Autodesk Inventor part; units mm, degrees
ref_plane "ip_st_1_XY" through (0, 0, 0) normal (1, 0, 0) x (0, 0, -1)
ref_plane "ip_st_1_YZ" through (0, 0, 0) normal (0, 0, -1) x (0, 1, 0)
ref_plane "ip_st_1_ZX" through (0, 0, 0) normal (0, 1, 0) x (1, 0, 0)
sketch "Sketch_1" plane through (0, 0, 0) normal (0, 0, 1) x (1, 0, 0)
  line L0 (4, 0) -> (0, 0)
  line L1 (0, 4.925) -> (0.25, 4.925)
  line L2 (0.25, 4.925) -> (0.25, 4.475)
  line L3 (0.25, 4.475) -> (1.2405, 4.475)
  arc A0 (2.7595, 4.475) -> (1.2405, 4.475) centre (2, 3.75) ccw
  line L4 (2.7595, 4.475) -> (3.75, 4.475)
  line L5 (3.75, 4.475) -> (3.75, 4.925)
  line L6 (3.75, 4.925) -> (4, 4.925)
  line L7 (4, 4.925) -> (4, 6.1)
  arc A1 (4, 6.1) -> (3.85, 6.25) centre (3.85, 6.1) ccw
  line L8 (3.85, 6.25) -> (3, 6.25)
  line L9 (3, 6.25) -> (3, 5.5)
  line L10 (3, 5.5) -> (0.15, 5.5)
  arc A2 (0.15, 5.5) -> (0, 5.35) centre (0.15, 5.35) ccw
  line L11 (0, 5.35) -> (0, 4.925)
revolve "Revolution1" add sketch "Sketch_1" angle 360 about axis through (4, 0, 0) along (1, 0, 0)
ref_plane "ip_st_1_XY" through (0, 0, 0) normal (1, 0, 0) x (0, 0, -1)
ref_plane "ip_st_1_YZ" through (0, 0, 0) normal (0, 0, -1) x (0, 1, 0)
ref_plane "ip_st_1_ZX" through (0, 0, 0) normal (0, 1, 0) x (1, 0, 0)
ref_plane "ip_st_2_XY" through (3.75, 0, 0) normal (-1, 0, 0) x (0, 0, -1)
ref_plane "ip_st_2_YZ" through (3.75, 0, 0) normal (0, 0, -1) x (0, -1, 0)
ref_plane "ip_st_2_ZX" through (3.75, 0, 0) normal (0, -1, 0) x (-1, 0, 0)
properties part number "F694ZZ Outer Ring" material "ステンレス鋼 440C"
For this review, take the finished solid that the model builds, in its own axes (mm). Coordinates: 2 decimals unless noted, no trailing zeros. Write each loop counter-clockwise with the first axis right and the second up, starting at its lowest first coordinate (ties: lowest second). Pieces come first, ordered by that corner, then holes. Notation, with made-up numbers: (13.25, 83) -> (61.25, 83) arc R17 cw to (61.25, 97) -> close; hole circle Ø9 at (25.5, 45). An arc over 180 degrees is marked (long way). Put each result on its own line as item: value.
Q1. Take a section at C-C, the plane x = 3.4. State the section outline as (y, z) points (3 decimals).
From the geometry:
outline: circle Ø12.5 at (0, 0); hole circle Ø8.95 at (0, 0)
Q2. Wall thickness on L1, parallel to Z at x = 0.15, y = 0 (3 decimals); L2, parallel to Z at x = 3.2, y = 0 (3 decimals); L3, parallel to X at y = 0.25, z = 4.5: over which ranges is each line inside the solid? List them lowest first.
From the geometry:
L1: z = -5.5 to -4.925, 4.925 to 5.5
L2: z = -6.25 to -4.475, 4.475 to 6.25
L3: x = 0.25 to 1.27, 2.73 to 3.75
Q3. The part is to be moulded in two halves that separate along Z. For faces 1 (the cylindrical face through (3.42, 5.96, -1.88)), 2 (the cylindrical face through (3.262, -3.551, -2.723)), 3 (the flat face through (3, 0, -6)), 4 (the cylindrical face through (0.752, -3.551, -2.723)), say which applies: +Z half, -Z half, draft (parallel to the pull), parting line (faces both ways), or undercut.
From the geometry:
face 1: parting line
face 2: undercut
face 3: draft
face 4: undercut
Q4. Take a section at D-D, the plane x = 0.65. State the section outline as (y, z) points (3 decimals).
From the geometry:
outline: circle Ø11 at (0, 0); hole circle Ø8.95 at (0, 0)
